```python
from build123d import *

# Parameters (mm, degrees)
F0_R     = 73.9775
F1_DEPTH = 21.59
F2_DEPTH = 21.59
F3_DEPTH = 43.18
F4_DEPTH = 76.2
F6_DEPTH = 25.4


with BuildPart() as f1:
    # F0 (on Front) → F1 (new body)
    with BuildSketch(Plane.XZ):
        Circle(F0_R)
        with BuildLine():
            ThreePointArc((9.4903436379, 55.0682102273), (21.3843502006, 51.6263882767), (32.2284185374, 45.6497912216))
            ThreePointArc((32.2284185374, 45.6497912216), (42.7795299647, 48.4605419914), (49.0381269327, 39.5131269327))
            ThreePointArc((49.0381269327, 39.5131269327), (48.1496005288, 35.4960448046), (45.6497912216, 32.2284185374))
            ThreePointArc((45.6497912216, 32.2284185374), (51.6263882767, 21.3843502006), (55.0682102273, 9.4903436379))
            ThreePointArc((55.0682102273, 9.4903436379), (62.3217904116, 7.0163353179), (65.405, 0))
            ThreePointArc((65.405, 0), (62.3217904116, -7.0163353179), (55.0682102273, -9.4903436379))
            ThreePointArc((55.0682102273, -9.4903436379), (51.6263882767, -21.3843502006), (45.6497912216, -32.2284185374))
            ThreePointArc((45.6497912216, -32.2284185374), (48.1496005288, -35.4960448046), (49.0381269327, -39.5131269327))
            ThreePointArc((49.0381269327, -39.5131269327), (42.7795299647, -48.4605419914), (32.2284185374, -45.6497912216))
            ThreePointArc((32.2284185374, -45.6497912216), (21.3843502006, -51.6263882767), (9.4903436379, -55.0682102273))
            ThreePointArc((9.4903436379, -55.0682102273), (9.5163319654, -55.4737354007), (9.525, -55.88))
            ThreePointArc((9.525, -55.88), (-0.4062645993, -65.3963319654), (-9.4903436379, -55.0682102273))
            ThreePointArc((-9.4903436379, -55.0682102273), (-21.3843502006, -51.6263882767), (-32.2284185374, -45.6497912216))
            ThreePointArc((-32.2284185374, -45.6497912216), (-46.2483190235, -46.2483190235), (-45.6497912216, -32.2284185374))
            ThreePointArc((-45.6497912216, -32.2284185374), (-51.6263882767, -21.3843502006), (-55.0682102273, -9.4903436379))
            ThreePointArc((-55.0682102273, -9.4903436379), (-65.405, 0), (-55.0682102273, 9.4903436379))
            ThreePointArc((-55.0682102273, 9.4903436379), (-51.6263882767, 21.3843502006), (-45.6497912216, 32.2284185374))
            ThreePointArc((-45.6497912216, 32.2284185374), (-46.2483190235, 46.2483190235), (-32.2284185374, 45.6497912216))
            ThreePointArc((-32.2284185374, 45.6497912216), (-21.3843502006, 51.6263882767), (-9.4903436379, 55.0682102273))
            ThreePointArc((-9.4903436379, 55.0682102273), (-0.4062645993, 65.3963319654), (9.525, 55.88))
            ThreePointArc((9.525, 55.88), (9.5163319654, 55.4737354007), (9.4903436379, 55.0682102273))
        make_face(mode=Mode.SUBTRACT)
    extrude(amount=F1_DEPTH)

    # F0 (on Front) → F2 (join)
    with BuildSketch(Plane.XZ):
        with BuildLine():
            ThreePointArc((-26.9407683632, -26.9407683632), (-38.1, 0), (-26.9407683632, 26.9407683632))
            Line((-26.9407683632, 26.9407683632), (-32.7779348419, 32.7779348419))
            ThreePointArc((-32.7779348419, 32.7779348419), (-39.1068623334, 29.9967949673), (-45.6497912216, 32.2284185374))
            ThreePointArc((-45.6497912216, 32.2284185374), (-51.6263882767, 21.3843502006), (-55.0682102273, 9.4903436379))
            ThreePointArc((-55.0682102273, 9.4903436379), (-48.8636646821, 6.4417904116), (-46.355, 0))
            ThreePointArc((-46.355, 0), (-48.8636646821, -6.4417904116), (-55.0682102273, -9.4903436379))
            ThreePointArc((-55.0682102273, -9.4903436379), (-51.6263882767, -21.3843502006), (-45.6497912216, -32.2284185374))
            ThreePointArc((-45.6497912216, -32.2284185374), (-39.1068623334, -29.9967949673), (-32.7779348419, -32.7779348419))
            Line((-32.7779348419, -32.7779348419), (-26.9407683632, -26.9407683632))
        make_face()
        with BuildLine():
            ThreePointArc((-26.9407683632, 26.9407683632), (0, 38.1), (26.9407683632, 26.9407683632))
            Line((26.9407683632, 26.9407683632), (32.7779348419, 32.7779348419))
            ThreePointArc((32.7779348419, 32.7779348419), (29.9967949673, 39.1068623334), (32.2284185374, 45.6497912216))
            ThreePointArc((32.2284185374, 45.6497912216), (21.3843502006, 51.6263882767), (9.4903436379, 55.0682102273))
            ThreePointArc((9.4903436379, 55.0682102273), (0, 46.355), (-9.4903436379, 55.0682102273))
            ThreePointArc((-9.4903436379, 55.0682102273), (-21.3843502006, 51.6263882767), (-32.2284185374, 45.6497912216))
            ThreePointArc((-32.2284185374, 45.6497912216), (-30.565711874, 42.7795299647), (-29.9881269327, 39.5131269327))
            ThreePointArc((-29.9881269327, 39.5131269327), (-30.7131743855, 35.8680672394), (-32.7779348419, 32.7779348419))
            Line((-32.7779348419, 32.7779348419), (-26.9407683632, 26.9407683632))
        make_face()
        with BuildLine():
            Line((32.7779348419, 32.7779348419), (26.9407683632, 26.9407683632))
            ThreePointArc((26.9407683632, 26.9407683632), (35.1998101887, 14.5802387731), (38.1, 0))
            ThreePointArc((38.1, 0), (35.1998101887, -14.5802387731), (26.9407683632, -26.9407683632))
            Line((26.9407683632, -26.9407683632), (32.7779348419, -32.7779348419))
            ThreePointArc((32.7779348419, -32.7779348419), (39.1068623334, -29.9967949673), (45.6497912216, -32.2284185374))
            ThreePointArc((45.6497912216, -32.2284185374), (51.6263882767, -21.3843502006), (55.0682102273, -9.4903436379))
            ThreePointArc((55.0682102273, -9.4903436379), (46.355, 0), (55.0682102273, 9.4903436379))
            ThreePointArc((55.0682102273, 9.4903436379), (51.6263882767, 21.3843502006), (45.6497912216, 32.2284185374))
            ThreePointArc((45.6497912216, 32.2284185374), (39.1068623334, 29.9967949673), (32.7779348419, 32.7779348419))
        make_face()
        with BuildLine():
            Line((32.7779348419, -32.7779348419), (26.9407683632, -26.9407683632))
            ThreePointArc((26.9407683632, -26.9407683632), (0, -38.1), (-26.9407683632, -26.9407683632))
            Line((-26.9407683632, -26.9407683632), (-32.7779348419, -32.7779348419))
            ThreePointArc((-32.7779348419, -32.7779348419), (-30.7131743855, -35.8680672394), (-29.9881269327, -39.5131269327))
            ThreePointArc((-29.9881269327, -39.5131269327), (-30.565711874, -42.7795299647), (-32.2284185374, -45.6497912216))
            ThreePointArc((-32.2284185374, -45.6497912216), (-21.3843502006, -51.6263882767), (-9.4903436379, -55.0682102273))
            ThreePointArc((-9.4903436379, -55.0682102273), (0, -46.355), (9.4903436379, -55.0682102273))
            ThreePointArc((9.4903436379, -55.0682102273), (21.3843502006, -51.6263882767), (32.2284185374, -45.6497912216))
            ThreePointArc((32.2284185374, -45.6497912216), (29.9967949673, -39.1068623334), (32.7779348419, -32.7779348419))
        make_face()
    extrude(amount=F2_DEPTH)

    # F0 (on Front) → F3 (join)
    with BuildSketch(Plane.XZ):
        with BuildLine():
            ThreePointArc((-15.7154482119, 15.7154482119), (0, 22.225), (15.7154482119, 15.7154482119))
            Line((15.7154482119, 15.7154482119), (26.9407683632, 26.9407683632))
            ThreePointArc((26.9407683632, 26.9407683632), (0, 38.1), (-26.9407683632, 26.9407683632))
            Line((-26.9407683632, 26.9407683632), (-15.7154482119, 15.7154482119))
        make_face()
        with BuildLine():
            Line((26.9407683632, 26.9407683632), (15.7154482119, 15.7154482119))
            ThreePointArc((15.7154482119, 15.7154482119), (20.5332226101, 8.5051392843), (22.225, 0))
            ThreePointArc((22.225, 0), (20.5332226101, -8.5051392843), (15.7154482119, -15.7154482119))
            Line((15.7154482119, -15.7154482119), (26.9407683632, -26.9407683632))
            ThreePointArc((26.9407683632, -26.9407683632), (35.1998101887, -14.5802387731), (38.1, 0))
            ThreePointArc((38.1, 0), (35.1998101887, 14.5802387731), (26.9407683632, 26.9407683632))
        make_face()
        with BuildLine():
            Line((26.9407683632, -26.9407683632), (15.7154482119, -15.7154482119))
            ThreePointArc((15.7154482119, -15.7154482119), (0, -22.225), (-15.7154482119, -15.7154482119))
            Line((-15.7154482119, -15.7154482119), (-26.9407683632, -26.9407683632))
            ThreePointArc((-26.9407683632, -26.9407683632), (0, -38.1), (26.9407683632, -26.9407683632))
        make_face()
        with BuildLine():
            ThreePointArc((-15.7154482119, -15.7154482119), (-22.225, 0), (-15.7154482119, 15.7154482119))
            Line((-15.7154482119, 15.7154482119), (-26.9407683632, 26.9407683632))
            ThreePointArc((-26.9407683632, 26.9407683632), (-38.1, 0), (-26.9407683632, -26.9407683632))
            Line((-26.9407683632, -26.9407683632), (-15.7154482119, -15.7154482119))
        make_face()
    extrude(amount=F3_DEPTH)

    # F0 (on Front) → F4 (join)
    with BuildSketch(Plane.XZ):
        with BuildLine():
            ThreePointArc((-8.9802561211, 8.9802561211), (0, 12.7), (8.9802561211, 8.9802561211))
            Line((8.9802561211, 8.9802561211), (15.7154482119, 15.7154482119))
            ThreePointArc((15.7154482119, 15.7154482119), (0, 22.225), (-15.7154482119, 15.7154482119))
            Line((-15.7154482119, 15.7154482119), (-8.9802561211, 8.9802561211))
        make_face()
        with BuildLine():
            ThreePointArc((8.9802561211, 8.9802561211), (11.7332700629, 4.860079591), (12.7, 0))
            ThreePointArc((12.7, 0), (11.7332700629, -4.860079591), (8.9802561211, -8.9802561211))
            Line((8.9802561211, -8.9802561211), (15.7154482119, -15.7154482119))
            ThreePointArc((15.7154482119, -15.7154482119), (20.5332226101, -8.5051392843), (22.225, 0))
            ThreePointArc((22.225, 0), (20.5332226101, 8.5051392843), (15.7154482119, 15.7154482119))
            Line((15.7154482119, 15.7154482119), (8.9802561211, 8.9802561211))
        make_face()
        with BuildLine():
            Line((15.7154482119, -15.7154482119), (8.9802561211, -8.9802561211))
            ThreePointArc((8.9802561211, -8.9802561211), (6.2997856733, -11.0273614464), (3.175, -12.2967221242))
            Line((3.175, -12.2967221242), (3.175, -15.875))
            Line((3.175, -15.875), (-3.175, -15.875))
            Line((-3.175, -15.875), (-3.175, -12.2967221242))
            ThreePointArc((-3.175, -12.2967221242), (-6.2997856733, -11.0273614464), (-8.9802561211, -8.9802561211))
            Line((-8.9802561211, -8.9802561211), (-15.7154482119, -15.7154482119))
            ThreePointArc((-15.7154482119, -15.7154482119), (0, -22.225), (15.7154482119, -15.7154482119))
        make_face()
        with BuildLine():
            ThreePointArc((-8.9802561211, -8.9802561211), (-12.7, 0), (-8.9802561211, 8.9802561211))
            Line((-8.9802561211, 8.9802561211), (-15.7154482119, 15.7154482119))
            ThreePointArc((-15.7154482119, 15.7154482119), (-22.225, 0), (-15.7154482119, -15.7154482119))
            Line((-15.7154482119, -15.7154482119), (-8.9802561211, -8.9802561211))
        make_face()
        with BuildLine():
            Line((3.175, -15.875), (3.175, -12.2967221242))
            ThreePointArc((3.175, -12.2967221242), (0, -12.7), (-3.175, -12.2967221242))
            Line((-3.175, -12.2967221242), (-3.175, -15.875))
            Line((-3.175, -15.875), (3.175, -15.875))
        make_face()
    extrude(amount=F4_DEPTH)

    # F5 (on face) → F6 (cut)
    with BuildSketch(Plane.XZ.offset(76.2)):
        with BuildLine():
            Line((-3.175, -15.875), (3.175, -15.875))
            Line((3.175, -15.875), (3.175, -12.2967221242))
            ThreePointArc((3.175, -12.2967221242), (0, -12.7), (-3.175, -12.2967221242))
            Line((-3.175, -12.2967221242), (-3.175, -15.875))
        make_face()
    extrude(amount=-F6_DEPTH, mode=Mode.SUBTRACT)


solid = f1.part
```
Check sheet for the modelled part. Datum: model origin and axes. Units: mm. A direction names the side the tool comes from. Coordinates: 2 decimals unless noted, no trailing zeros. Order: outer loops, then holes, each group sorted by start corner. A loop starts at its lowest first (then second) coordinate and runs counter-clockwise, first axis right, second up. Notation, with made-up numbers: (-39.75, 11.25) -> (6.25, 11.25) arc R33 ccw to (6.25, 50.25) -> close; hole circle Ø8 at (36, -29.5). An arc over 180 degrees is marked (long way). Write item = value, one per line. Start each with the question number.
1) Go/stop test with flat-tipped pins: P1, Ø12, axis at x = -37, y = -27, coming from the +Z side; P2, Ø4, axis at y = -31, z = -31, coming from the -X side; P3, Ø7, axis at x = 0, y = -60, coming from the +Z side (3 decimals). Record where each tip stops, or that it passes through.
2) Material ranges on L1, parallel to Z at x = -0.5, y = -33; L2, parallel to Z at x = -0.5, y = -50; L3, parallel to Z at x = 44, y = -13.5, recorded low to high.
3) Cross-section at D-D (x = -57.5). Enter the section's corners in (y, z).
4) Cross-section at C-C (z = 59). Enter the section's corners in (x, y), then the cut area to 3 significant figures.
5) Access from +Z, -Z, +X, -X, +Y, -Y to the whole of each face (thin tool, end or side, straight path). Record for faces 5 (the flat face through (32, -21.59, -32)), 6 (the flat face through (10, -76.2, -10)).
6) Cross-section at B-B (y = -29). Enter the section's corners in (x, z) (3 decimals).
7) Mould release check, pull along Z, two halves, no side actions. Record for faces 1 (the flat face through (-3.175, -64, -14)), 2 (the flat face through (0, -50.8, -14)), 3 (the cylindrical face through (-16.037, -10.644, -72.218)), 4 (the flat face through (15, 0, 1)): +Z half, -Z half, draft (parallel to the pull), parting line (faces both ways), or undercut.
8) Cross-section at A-A (x = 0). Enter the section's corners in (y, z) (1 decimal), then the cut area to 3 significant figures.
Ans:
q1.P1 = 65.49
q1.P2 = -24.71
q1.P3 = 22.225
q2.L1 = -38.1 to -12.69, 12.69 to 38.1
q2.L2 = -22.22 to -12.69, 12.69 to 22.22
q2.L3 = -59.47 to -47.92, -31.11 to 31.11, 47.92 to 59.47
q3.outline = (-21.59, -46.54) -> (0, -46.54) -> (0, -9.39) -> (-21.59, -9.39) -> close; (-21.59, 9.39) -> (0, 9.39) -> (0, 46.54) -> (-21.59, 46.54) -> close
q4.outline = (-44.63, -21.59) -> (-9, -21.59) -> (-9, 0) -> (-44.63, 0) -> close; (9, -21.59) -> (44.63, -21.59) -> (44.63, 0) -> (9, 0) -> close
q4.area = 1,540 mm²
q5.face_5 = -Y
q5.face_6 = +Z, -Z, +X, -X, -Y
q6.outline = circle Ø76.2 at (0, 0); hole circle Ø25.4 at (0, 0)
q7.face_1 = undercut
q7.face_2 = undercut
q7.face_3 = parting line
q7.face_4 = draft
q8.outline = (-76.2, -22.2) -> (-43.2, -22.2) -> (-43.2, -38.1) -> (-21.6, -38.1) -> (-21.6, -46.4) -> (0, -46.4) -> (0, -12.7) -> (-50.8, -12.7) -> (-50.8, -15.9) -> (-76.2, -15.9) -> close; (-76.2, 12.7) -> (0, 12.7) -> (0, 46.4) -> (-21.6, 46.4) -> (-21.6, 38.1) -> (-43.2, 38.1) -> (-43.2, 22.2) -> (-76.2, 22.2) -> close; (-21.6, -74) -> (0, -74) -> (0, -65.4) -> (-21.6, -65.4) -> close; (-21.6, 65.4) -> (0, 65.4) -> (0, 74) -> (-21.6, 74) -> close
q8.area = 3,470 mm²
